from build123d import *

# Parameters (mm, degrees)
F1_DEPTH    = 22
F2_DEPTH    = 17
F3_T4_DEPTH = 49.7168298797
F5_DEPTH    = 44
F0_W        = 11
F0_H        = 4
F6_DEPTH    = 15
F7_W        = 11
F7_H        = 2.2102209181
F8_DEPTH    = 14
F9_R        = 14
F9_R_2      = 12.5
F10_DEPTH   = 13
F12_R       = 0.5


# Not quite as in the source:
# - a fillet or chamfer that OpenCascade refuses, or shapes differently, is made with other operations: its cross-section is extruded or revolved along the edge and cut away or added


with BuildPart() as f1:
    # F0 (on Top) → F1 (new body)
    with BuildSketch(Plane.XY):
        Polygon((22, 9), (22, 22), (5.5, 22), (5.5, 18), (-5.5, 18), (-5.5, 22), (-22, 22), (-22, 9), (-18, 4), (-18, -4), (-22, -9), (-22, -22), (-12, -22), (-7, -19), (7, -19), (12, -22), (22, -22), (22, -9), (18, -4), (18, 4), align=None)
    extrude(amount=F1_DEPTH)

    # F0 (on Top) → F2 (join)
    with BuildSketch(Plane.XY):
        Polygon((-12, -22), (12, -22), (7, -19), (-7, -19), align=None)
    extrude(amount=F2_DEPTH)

    # F3: chamfer of 5 on 1 edges, made by hand


with BuildPart() as f3_tool2:
    # F3_s3 → F3_t4 (new body)
    with BuildSketch(Plane.YZ.offset(-24.8584149398)):
        Polygon((-17, 17), (-22, 12), (-22, 17), align=None)
    extrude(amount=F3_T4_DEPTH)

    split(bisect_by=Plane(origin=(-6.5294117647, -10.8823529412, 0), x_dir=(0, 0, 1), z_dir=(-0.5144957554, -0.8574929257, 0)), keep=Keep.TOP)

    split(bisect_by=Plane.XZ.offset(19), keep=Keep.TOP)

    split(bisect_by=Plane(origin=(6.5294117647, -10.8823529412, 0), x_dir=(0, 0, 1), z_dir=(0.5144957554, -0.8574929257, 0)), keep=Keep.TOP)


with BuildPart() as f1_1:
    add(f1.part)

    # F3_t1: cut F3_tool2
    add(f3_tool2.part, mode=Mode.SUBTRACT)

    # F4 (on face) → F5 (cut, through all)
    with BuildSketch(Plane.YZ.offset(22)):
        Polygon((8.5, 8), (-8.5, 8), (-8.5, 0), (0, 0), (8.5, 0), align=None)
    extrude(amount=-F5_DEPTH, mode=Mode.SUBTRACT)

    # F0 (on Top) → F6 (join)
    with BuildSketch(Plane.XY):
        with Locations((0, 20)):
            Rectangle(F0_W, F0_H)
    extrude(amount=F6_DEPTH)

    # F7 (on face) → F8 (join)
    with BuildSketch(Plane(origin=(0, 18, 0), x_dir=(-1, 0, 0), z_dir=(0, 1, 0))):
        with Locations((0, 16.105110459)):
            Rectangle(F7_W, F7_H)
    extrude(amount=F8_DEPTH)

    # F9 (on face) → F10 (join)
    with BuildSketch(Plane.XY.offset(22)):
        Circle(F9_R)
        Circle(F9_R_2, mode=Mode.SUBTRACT)
    extrude(amount=F10_DEPTH)

    # F11: fillet of radius 5 on 1 edges, made by hand

    # F11_s1 → F11_t2 (revolve, cut)
    with BuildSketch(Plane.XZ):
        with BuildLine():
            ThreePointArc((14, 35), (12.8902277714, 33.3657774588), (12.5, 31.4292857857))
            Line((12.5, 31.4292857857), (12.5, 35))
            Line((12.5, 35), (14, 35))
        make_face()
    revolve(axis=Axis((0, 0, 35), (0, 0, 1)), mode=Mode.SUBTRACT)

    # F12
    f12_edges = [f1_1.edges().sort_by_distance(p)[0] for p in [
        (22, 15.5, 22),
        (20, 6.5, 22),
        (13.75, 22, 22),
        (18, 0, 22),
        (5.5, 20, 22),
        (20, -6.5, 22),
        (0, 18, 22),
        (22, -15.5, 22),
        (-5.5, 20, 22),
        (17, -22, 22),
        (-13.75, 22, 22),
        (9.5, -20.5, 22),
        (-22, 15.5, 22),
        (0, -19, 22),
        (-20, 6.5, 22),
        (-9.5, -20.5, 22),
        (-18, 0, 22),
        (-17, -22, 22),
        (-20, -6.5, 22),
        (-22, -15.5, 22),
        (-14, 0, 22),
        (21.8, 8.75, 0),
        (22, 15.5, 0),
        (0, 22, 0),
        (-22, 15.5, 0),
        (-21.8, 8.75, 0),
        (0, 8.5, 0),
        (21.8, -8.75, 0),
        (22, -15.5, 0),
        (0, -22, 0),
        (-22, -15.5, 0),
        (-21.8, -8.75, 0),
        (0, -8.5, 0),
        (7, -19, 18.5),
        (0, -19, 15),
        (-7, -19, 18.5),
        (-22, -22, 11),
        (-12, -22, 17),
        (0, -22, 12),
        (12, -22, 17),
        (22, -22, 11),
        (-22, -9, 11),
    ]]
    fillet(f12_edges, radius=F12_R)


solid = f1_1.part
The listing builds one solid part. Answer for the finished solid, in the listing's coordinates (mm). A direction names the side the tool comes from. Round coordinates to 2 decimals unless told otherwise and drop trailing zeros. Loops run counter-clockwise (first coordinate to the right, second up) from the corner with the lowest first, then second, coordinate; pieces in that order, holes last. Notation, with made-up numbers: M 88,4 L 146,4 A20 ccw 146,18 Z; hole C 0,86 d6. An arc over 180 degrees is marked long. Write each question's results on one line, items separated by ' | '. Start each with the question number.
1) Which of the six approach directions +Z, -Z, +X, -X, +Y, -Y give full straight-line access (tool end or side, diameter ignored) to faces 1 (the cylindrical face through (12.932, -5.362, 28.662)), 2 (the cylindrical face through (9.61, -20.39, 21.86)), 3 (the flat face through (20, 6.5, 13.2)), 4 (the flat face through (5.5, 27, 16)), 5 (the flat face through (0, 27, 15))?
2) Find section A-A on z = 3.5. Write down the section's boundary in (x, y).
3) Find section D-D on y = 0. Write down the section's boundary in (x, z).
4) Determine the mould class of faces 6 (the flat face through (0, 18, 19)), 7 (the flat face through (18, 0, 15)), 8 (the flat face through (0, -22, 9)), 9 (the flat face through (0, 0, 22)) for opening direction X: pulls with the +X half, pulls with the -X half, needs draft (parallel to the pull), parting line crosses it, or undercut.
5) Straight lines are drawn through the part: probe 1 along Y at (x, z) = (0, 28); probe 2 along Z at (x, y) = (8, 17); probe 3 along Z at (x, y) = (-17.5, -7). For each, find the intervals that lie inside material, in ascending order.
6) Each of these flat-tipped pins is pushed along its axis until it touches: pin 1 (2 mm diameter, centred on x = 10.5, z = 4, fed in from +Y); pin 2 (4 mm diameter, centred on y = 0, z = 13, fed in from +X); pin 3 (2 mm diameter, centred on x = 11, z = 30, fed in from +Y). Where does it stop, or does it pass through?
7) Find section C-C on z = 20. Write down the section's boundary in (x, y).
Final values:
1) face 1: +Z | face 2: +Z, -Y | face 3: +Z, -Z, +X | face 4: +Z, -Z, +X, +Y | face 5: -Z, +X, -X, +Y
2) outline: M -22,-21.5 A0.5 ccw -21.5,-22 L 21.5,-22 A0.5 ccw 22,-21.5 L 22,-9 L 21.6,-8.5 L -21.6,-8.5 L -21.89,-8.86 A0.5 ccw -22,-9.18 Z; M -22,9 L -21.6,8.5 L 21.6,8.5 L 22,9 L 22,22 L -22,22 Z
3) outline: M -18,8 L 18,8 L 18,21.5 A0.5 ccw 17.5,22 L 14.5,22 A0.5 cw 14,22.5 L 14,35 A5 ccw 12.5,31.43 L 12.5,22 L -12.5,22 L -12.5,31.43 A5 ccw -14,35 L -14,22.5 A0.5 cw -14.5,22 L -17.5,22 A0.5 ccw -18,21.5 Z
4) face 6: undercut | face 7: pulls with the +X half | face 8: needs draft | face 9: undercut
5) probe 1: -14 to -12.5, 12.5 to 14 | probe 2: 0 to 22 | probe 3: 8 to 22
6) pin 1: y = 22 | pin 2: x = 18 | pin 3: y = 9.8
7) outline: M -22,-21.5 A0.5 ccw -21.5,-22 L -12.14,-22 A0.5 ccw -11.88,-21.93 L -7.12,-19.07 A0.5 cw -6.86,-19 L 6.86,-19 A0.5 cw 7.12,-19.07 L 11.88,-21.93 A0.5 ccw 12.14,-22 L 21.5,-22 A0.5 ccw 22,-21.5 L 22,-9 L 18,-4 L 18,4 L 22,9 L 22,22 L 5.5,22 L 5.5,18 L -5.5,18 L -5.5,22 L -22,22 L -22,9 L -18,4 L -18,-4 L -21.89,-8.86 A0.5 ccw -22,-9.18 Z
